Part model, mm, in its own coordinate system. Face numbers are marked on the shaded views. A direction names the side the tool comes from. Give positions to 0.01 mm unless a question says otherwise; leave off trailing zeros. Write each loop counter-clockwise with the first axis right and the second up, starting at its lowest first coordinate (ties: lowest second). Pieces come first, ordered by that corner, then holes. Notation, with made-up numbers: M 67,-7.5 L 74,-7.5 A18 cw 74,14.5 Z; hole C 49.25,38 d8. An arc over 180 degrees is marked long. Use a Markdown table: item, result.
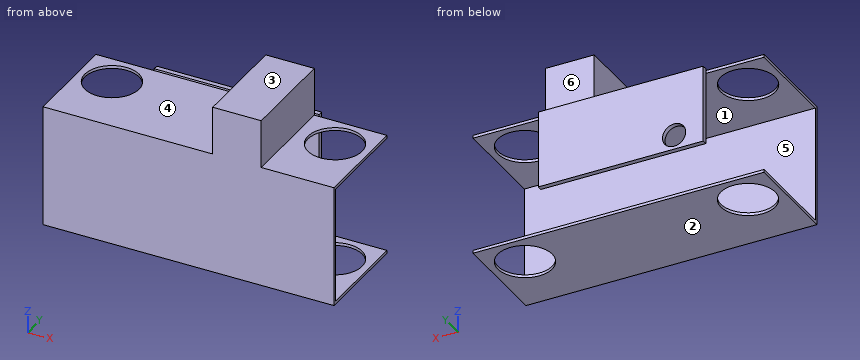
```python
from build123d import *

# Parameters (mm, degrees)
SKETCH1_W            = 300
SKETCH1_H            = 126
BOSS_EXTRUDE2_DEPTH  = 3
SKETCH3_W            = 300
SKETCH3_H            = 3
BOSS_EXTRUDE3_DEPTH  = 100
SKETCH4_R            = 28
CUT_EXTRUDE1_DEPTH   = 186
SKETCH5_W            = 50
SKETCH5_H            = 103
BOSS_EXTRUDE9_DEPTH  = 50
SKETCH9_W            = 170
SKETCH9_H            = 80
SKETCH9_R            = 12
BOSS_EXTRUDE14_DEPTH = 5


with BuildPart() as part:
    # Sketch1 → Boss-Extrude2 (new body)
    with BuildSketch(Plane(origin=(0, 0, 0), x_dir=(1, 0, 0), z_dir=(0, 1, 0))):
        with Locations((3.935860058, -11.344023324)):
            Rectangle(SKETCH1_W, SKETCH1_H)
    extrude(amount=BOSS_EXTRUDE2_DEPTH)

    # Sketch3 → Boss-Extrude3 (add)
    with BuildSketch(Plane(origin=(0, 3, 0), x_dir=(1, 0, 0), z_dir=(0, 1, 0))):
        with Locations((3.935860058, -72.844023324)):
            Rectangle(SKETCH3_W, SKETCH3_H)
        with Locations((3.935860058, 50.155976676)):
            Rectangle(SKETCH3_W, SKETCH3_H)
    extrude(amount=BOSS_EXTRUDE3_DEPTH)

    # Sketch4 → Cut-Extrude1 (cut)
    with BuildSketch(Plane.XY.offset(74.344023324)):
        with Locations((-111.064139942, 68)):
            Circle(SKETCH4_R)
        with Locations((118.935860058, 68)):
            Circle(SKETCH4_R)
    extrude(amount=-CUT_EXTRUDE1_DEPTH, mode=Mode.SUBTRACT)

    # Sketch5 → Boss-Extrude9 (add)
    with BuildSketch(Plane.XY.offset(74.344023324)):
        with Locations((53.935860058, 51.5)):
            Rectangle(SKETCH5_W, SKETCH5_H)
    extrude(amount=BOSS_EXTRUDE9_DEPTH)

    # Sketch9 → Boss-Extrude14 (add)
    with BuildSketch(Plane(origin=(0, 103, 0), x_dir=(1, 0, 0), z_dir=(0, 1, 0))):
        with Locations((-1.064139942, -36.344023324)):
            Rectangle(SKETCH9_W, SKETCH9_H)
        with Locations(Location((-56.064139942, -11.344023324, 0), (0, 0, 270))):
            Circle(SKETCH9_R, mode=Mode.SUBTRACT)
    extrude(amount=BOSS_EXTRUDE14_DEPTH)


solid = part.part
```
1. Drill centre lines: L1, parallel to Z at x = -100.5, y = 25.5; L2, parallel to Y at x = 76, z = 53; L3, parallel to Y at x = 124.5, z = 15.5. Where is each one in solid material? Low to high.
Findings below:
| item | result |
|---|---|
| L1 | -51.66 to -48.66, 71.34 to 74.34 |
| L2 | 0 to 3, 103 to 108 |
| L3 | 0 to 3 |
2. Two-plate mould, pull along Z, no slides. Class the marked faces 1, 2 and 3: released by +Z, released by -Z, zero draft, split by the parting line, or undercut.
Findings below:
| item | result |
|---|---|
| face 1 | undercut |
| face 2 | released by -Z |
| face 3 | released by +Z |
3. Tool access for the marked faces 4, 5 and 6: list every direction of +Z, -Z, +X, -X, +Y, -Y with a clear straight run to the whole face (end or side of a thin tool).
Findings below:
| item | result |
|---|---|
| face 4 | +Z, -X, -Y |
| face 5 | +X, -X |
| face 6 | +Z, +X, -X, +Y |
4. Cut at B-B, the plane z = 38.5. Give the cut face in (x, y), then the cut area to 3 significant figures.
Findings below:
| item | result |
|---|---|
| outline | M -146.06,0 L 153.94,0 L 153.94,3 L -146.06,3 Z; M -86.06,103 L 83.94,103 L 83.94,108 L -86.06,108 Z |
| area | 1,750 mm2 |
5. Drop flat-ended pins along their axis: P1, Ø1.5, axis at x = -33.5, y = 105, coming from the +Z side; P2, Ø1.5, axis at x = -130, z = 72, coming from the +Y side; P3, Ø1.5, axis at x = -42, y = 106.5, coming from the -Z side. Give the stop position or say it passes through.
Findings below:
| item | result |
|---|---|
| P1 | z = 76.34 |
| P2 | y = 103 |
| P3 | z = -3.66 |
6. Cut at C-C, the plane x = 103. Give the cut face in (y, z), then the cut area to 3 significant figures.
Findings below:
| item | result |
|---|---|
| outline | M 0,-51.66 L 44.98,-51.66 L 44.98,-48.66 L 3,-48.66 L 3,71.34 L 44.98,71.34 L 44.98,74.34 L 0,74.34 Z; M 91.02,-51.66 L 103,-51.66 L 103,-48.66 L 91.02,-48.66 Z; M 91.02,71.34 L 103,71.34 L 103,74.34 L 91.02,74.34 Z |
| area | 702 mm2 |
7. Cut at A-A, the plane y = 68. Give the cut face in (x, z).
Findings below:
| item | result |
|---|---|
| outline | M -146.06,-51.66 L -139.06,-51.66 L -139.06,-48.66 L -146.06,-48.66 Z; M -146.06,71.34 L -139.06,71.34 L -139.06,74.34 L -146.06,74.34 Z; M -83.06,-51.66 L 90.94,-51.66 L 90.94,-48.66 L -83.06,-48.66 Z; M -83.06,71.34 L 90.94,71.34 L 90.94,74.34 L 78.94,74.34 L 78.94,124.34 L 28.94,124.34 L 28.94,74.34 L -83.06,74.34 Z; M 146.94,-51.66 L 153.94,-51.66 L 153.94,-48.66 L 146.94,-48.66 Z; M 146.94,71.34 L 153.94,71.34 L 153.94,74.34 L 146.94,74.34 Z |
8. Cut at D-D, the plane z = 5. Give the cut face in (x, y), then the cut area to 3 significant figures.
Findings below:
| item | result |
|---|---|
| outline | M -146.06,0 L 153.94,0 L 153.94,3 L -146.06,3 Z; M -86.06,103 L -66.25,103 L -66.25,108 L -86.06,108 Z; M -45.88,103 L 83.94,103 L 83.94,108 L -45.88,108 Z |
| area | 1,650 mm2 |
